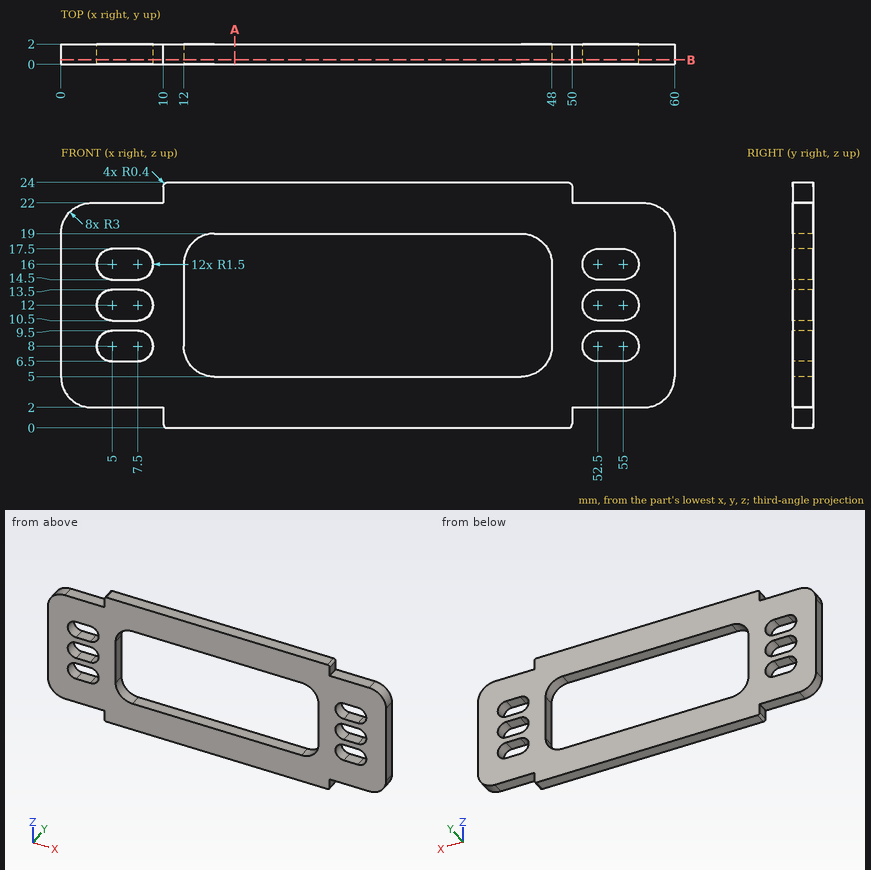
Answer from the drawing. Dimensions are ordinates in mm from the lowest x, y and z of the part. Coordinates: 2 decimals unless noted, no trailing zeros. Write each loop counter-clockwise with the first axis right and the second up, starting at its lowest first coordinate (ties: lowest second). Pieces come first, ordered by that corner, then holes. Notation, with made-up numbers: M -12.75,8 L 25.25,8 A31 cw 25.25,38 Z; hole C 17.5,-37.75 d7. An arc over 180 degrees is marked long. Use one line per item in the form item = value. Start each with the question number.
1. Straight lines are drawn through the part: probe 1 along Z at (x, y) = (37, 1.4); probe 2 along Z at (x, y) = (5, 1.9); probe 3 along X at (y, z) = (0.8, 8.5). For each, find the intervals that lie inside material, in ascending order. Write a range as from..to.
2. The part is cut by section B-B (y = 0.45). Give the number of separate pieces and of enclosed holes in the cut face, plus the area to 3 significant figures.
3. Each of these flat-tipped pins is pushed along its axis until it touches: P1, Ø1, axis at x = 7, y = 1, coming from the +Z side; P2, Ø0.6, axis at x = 53, y = 1.5, coming from the -Z side; P3, Ø10, axis at x = 39.5, z = 13.5, coming from the -Y side. Where does it stop, or does it pass through?
4. The part is cut by section A-A (x = 17). Give the vertices of the cut face in (y, z), plus the area to 3 significant figures.
Evaluation:
q1.probe_1 = 0..5, 19..24
q1.probe_2 = 2..6.5, 9.5..10.5, 13.5..14.5, 17.5..22
q1.probe_3 = 0..3.59, 8.91..12, 48..51.09, 56.41..60
q2.separate_pieces = 1
q2.enclosed_holes = 7
q2.area = 768 mm^2
q3.P1 = 22
q3.P2 = 2
q3.P3 = through
q4.outline = M 0,0 L 2,0 L 2,5 L 0,5 Z; M 0,19 L 2,19 L 2,24 L 0,24 Z
q4.area = 20.0 mm^2
